Read the model definition and answer for the solid it produces. Units are mm, in the model's axes. Face numbers are marked on the shaded views. A direction names the side the tool comes from. Round coordinates to 2 decimals unless told otherwise and drop trailing zeros. Order: outer loops, then holes, each group sorted by start corner. A loop starts at its lowest first (then second) coordinate and runs counter-clockwise, first axis right, second up. Notation, with made-up numbers: (-10.75, 65) - (32.25, 65) arc R15 cw to (32.25, 85) - close; hole circle Ø1 at (89.25, 67). An arc over 180 degrees is marked (long way). Put each result on its own line as item: value. Start each with the question number.
Q1. Section A-A on z = 0 is taken. State how many separate pieces and enclosed holes the cut face has, then the cut area to 3 significant figures.
Q2. Each of these flat-tipped pins is pushed along its axis until it touches: pin 1 Ø16.5 at (y, z) = (-26.99, 0) entering from -X; pin 2 Ø12.5 at (x, z) = (-42.5, -3.5) entering from -Y; pin 3 Ø23 at (x, z) = (-82.55, 0) entering from -Y; pin 4 Ø3 at (y, z) = (-103.5, 16) entering from +X. Where does it stop, or does it pass through?
Q3. Which of the six approach directions +Z, -Z, +X, -X, +Y, -Y give full straight-line access (tool end or side, diameter ignored) to the marked faces 4 and 5?
Q4. For a pull along Y with two mould halves and no side action, classify the marked faces 1, 2 and 3 as pulls with the +Y half, pulls with the -Y half, needs draft (parallel to the pull), parting line crosses it, or undercut.
Q5. Section B-B on x = -9.5 is taken. Give the vertices of the cut face in (y, z) (3 decimals).
Q6. Find the intervals of material crossed by line 1 along X through (y, z) = (-54.5, 11.5); line 2 along Y through (x, z) = (-37.5, -11); line 3 along X through (y, z) = (-20, 7.5), in increasing order. Write a range as from..to.
Q7. Section D-D on y = -87.5 is taken. Give the vertices of the cut face in (x, z) (1 decimal), then the cut area to 3 significant figures.
from build123d import *

# Parameters (mm, degrees)
EXTRUDE_THIN1_DEPTH = 20.574
BOSS_EXTRUDE1_DEPTH = 9.525
SKETCH3_R           = 7.112
CUT_EXTRUDE1_DEPTH  = 6.35
SKETCH4_R           = 7.112
CUT_EXTRUDE2_DEPTH  = 6.35


with BuildPart() as part:
    # Sketch1 → Extrude-Thin1 (new, symmetric)
    with BuildSketch(Plane.XY):
        with BuildLine():
            Line((-112.7125, -101.6), (-112.7125, -9.525))
            ThreePointArc((-112.7125, -9.525), (-109.922692091, -2.789807909), (-103.1875, 0))
            Line((-103.1875, 0), (103.1875, 0))
            Line((103.1875, 0), (103.1875, -6.35))
            Line((103.1875, -6.35), (-103.1875, -6.35))
            ThreePointArc((-103.1875, -6.35), (-105.43256403, -7.27993597), (-106.3625, -9.525))
            Line((-106.3625, -9.525), (-106.3625, -101.6))
            Line((-106.3625, -101.6), (-112.7125, -101.6))
        make_face()
    extrude(amount=EXTRUDE_THIN1_DEPTH, both=True)

    # Sketch2 → Boss-Extrude1 (add, symmetric)
    with BuildSketch(Plane.XY):
        Polygon((19.567609966, -6.35), (-106.3625, -101.6), (-112.7125, -101.6), (-112.7125, -106.402961739), (-122.2375, -113.607404348), (-118.406878416, -118.671872561), (30.093969492, -6.35), align=None)
    extrude(amount=BOSS_EXTRUDE1_DEPTH, both=True)

    # Sketch3 → Cut-Extrude1 (cut)
    with BuildSketch(Plane(origin=(0, 0, 0), x_dir=(1, 0, 0), z_dir=(0, 1, 0))):
        with Locations(Location((-82.55, 0, 0), (0, 0, 180))):
            Circle(SKETCH3_R)
        with Locations(Location((73.025, 0, 0), (0, 0, 180))):
            Circle(SKETCH3_R)
    extrude(amount=-CUT_EXTRUDE1_DEPTH, mode=Mode.SUBTRACT)

    # Sketch4 → Cut-Extrude2 (cut)
    with BuildSketch(Plane.ZY.offset(112.7125)):
        with Locations((0, -26.9875)):
            Circle(SKETCH4_R)
    extrude(amount=-CUT_EXTRUDE2_DEPTH, mode=Mode.SUBTRACT)


solid = part.part
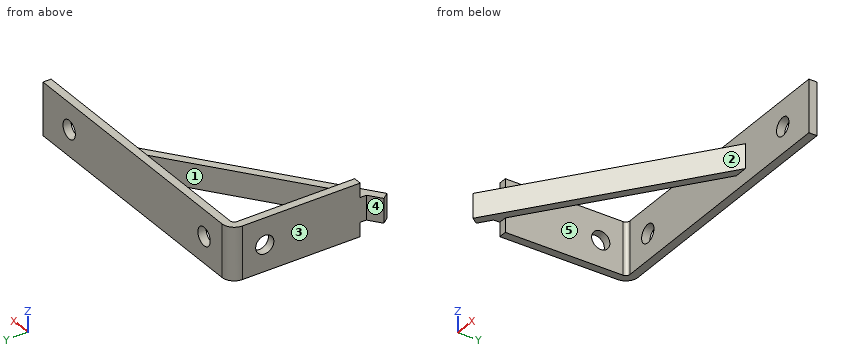
Findings:
1. separate pieces: 3
1. enclosed holes: 0
1. area: 2,860 mm2
2. pin 1: x = -112.71
2. pin 2: y = -65.99
2. pin 3: y = -100.25
2. pin 4: through
3. face 4: +Z, -Z, -X, +Y
3. face 5: +Z, -Z
4. face 1: undercut
4. face 2: pulls with the -Y half
4. face 3: needs draft
5. outline: (-36.298, -9.525) - (-28.336, -9.525) - (-28.336, 9.525) - (-36.298, 9.525) - close; (-6.35, -20.574) - (0, -20.574) - (0, 20.574) - (-6.35, 20.574) - close
6. line 1: -112.71..-106.36
6. line 2: -6.35..0
6. line 3: -112.71..-106.36, 1.52..12.05
7. outline: (-112.7, -20.6) - (-106.4, -20.6) - (-106.4, 20.6) - (-112.7, 20.6) - close; (-87.7, -9.5) - (-77.2, -9.5) - (-77.2, 9.5) - (-87.7, 9.5) - close
7. area: 462 mm2
